Verification items for this drawing (mm, ordinates from the low corner). A direction names the side the tool comes from. Round coordinates to 2 decimals unless told otherwise and drop trailing zeros. Order: outer loops, then holes, each group sorted by start corner. A loop starts at its lowest first (then second) coordinate and runs counter-clockwise, first axis right, second up. Notation, with made-up numbers: (76.5, -6.75) - (120.5, -6.75) arc R20 ccw to (120.5, -1.75) - close; hole circle Ø7 at (52.5, 10). An arc over 180 degrees is marked (long way). Return JSON: item names as keys, results as strings. Group by question number.
Q1. Sectioned sample at C-C, the plane y = 41. Record the cut outline in (x, z).
Q2. Material ranges on line 1 along X through (y, z) = (59.5, 19); line 2 along Z through (x, y) = (6.5, 19.5), recorded low to high.
Q3. Sectioned sample at D-D, the plane y = 27. Record the cut outline in (x, z), then the cut area to 3 significant figures.
Q4. Gauge pin test, flat ends, axial feed: pin 1 Ø5 at (y, z) = (50.8, 19) entering from -X; pin 2 Ø11.5 at (x, y) = (14, 23.5) entering from +Z; pin 3 Ø8.5 at (x, z) = (34, 5.5) entering from +Y; pin 4 Ø0.8 at (x, y) = (0.5, 55.5) entering from -Z. Record the tip position at first contact, or that the pin passes through.
Q5. Sectioned sample at A-A, the plane y = 50.8. Record the cut outline in (x, z), then the cut area to 3 significant figures.
Q6. Draft check along X on the marked faces 3, 4 and 5. Enter one of: pulls with the +X half, pulls with the -X half, needs draft (parallel to the pull), parting line crosses it, or undercut.
Q7. Sectioned sample at B-B, the plane z = 7. Record the cut outline in (x, y).
Q8. Tool access check on the marked faces 1 and 2. Record the directions out of +Z, -Z, +X, -X, +Y, -Y that give a thin tool (end or side, any length) a straight path to the whole face; none if there is none.
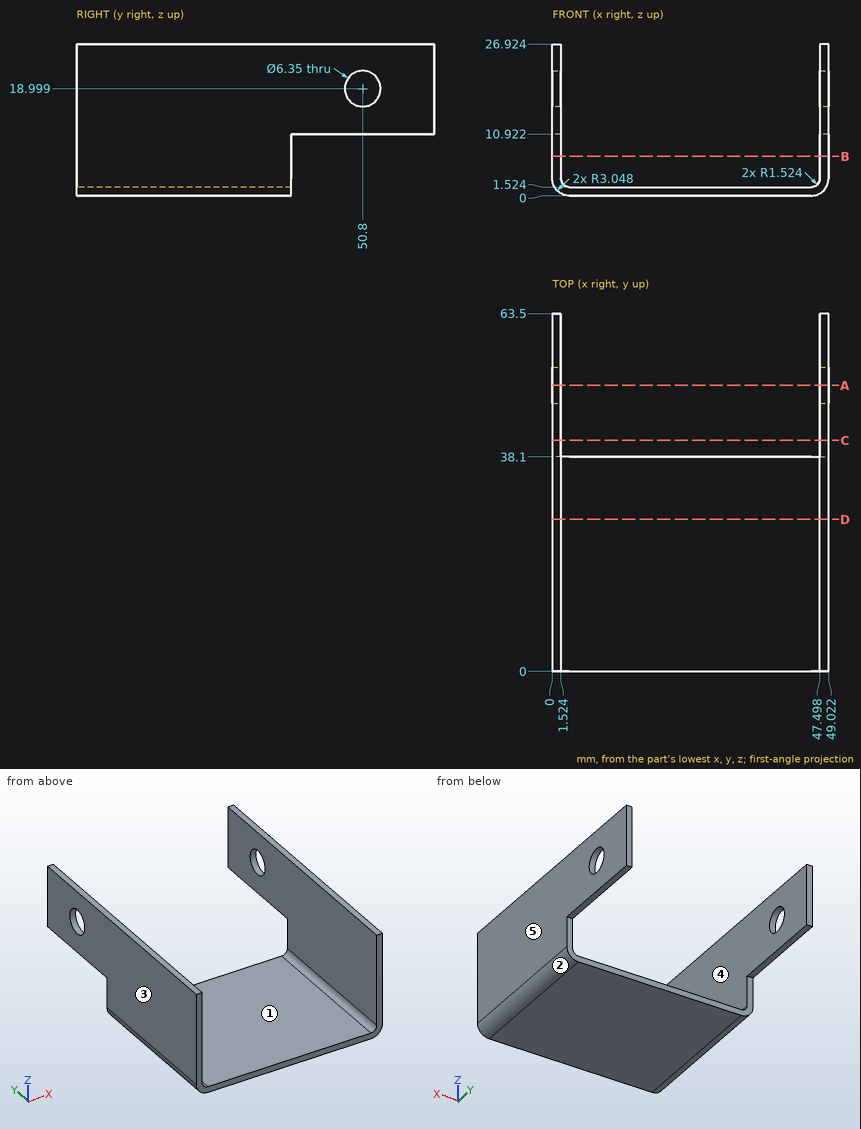
Reply:
{
 "1": {"outline": "(0, 10.92) - (1.52, 10.92) - (1.52, 26.92) - (0, 26.92) - close; (47.5, 10.92) - (49.02, 10.92) - (49.02, 26.92) - (47.5, 26.92) - close"},
 "2": {"line 1": "0 to 1.52, 47.5 to 49.02", "line 2": "0 to 1.52"},
 "3": {"outline": "(0, 3.05) arc R3.05 ccw to (3.05, 0) - (45.97, 0) arc R3.05 ccw to (49.02, 3.05) - (49.02, 26.92) - (47.5, 26.92) - (47.5, 3.05) arc R1.52 cw to (45.97, 1.52) - (3.05, 1.52) arc R1.52 cw to (1.52, 3.05) - (1.52, 26.92) - (0, 26.92) - close", "area": "149 mm^2"},
 "4": {"pin 1": "through", "pin 2": "z = 1.52", "pin 3": "y = 38.1", "pin 4": "z = 10.92"},
 "5": {"outline": "(0, 10.92) - (1.52, 10.92) - (1.52, 15.82) - (0, 15.82) - close; (0, 22.17) - (1.52, 22.17) - (1.52, 26.92) - (0, 26.92) - close; (47.5, 10.92) - (49.02, 10.92) - (49.02, 15.82) - (47.5, 15.82) - close; (47.5, 22.17) - (49.02, 22.17) - (49.02, 26.92) - (47.5, 26.92) - close", "area": "29.4 mm^2"},
 "6": {"face 3": "pulls with the -X half", "face 4": "undercut", "face 5": "pulls with the +X half"},
 "7": {"outline": "(0, 0) - (1.52, 0) - (1.52, 38.1) - (0, 38.1) - close; (47.5, 0) - (49.02, 0) - (49.02, 38.1) - (47.5, 38.1) - close"},
 "8": {"face 1": "+Z, +Y, -Y", "face 2": "-Z, +X, +Y, -Y"}
}
